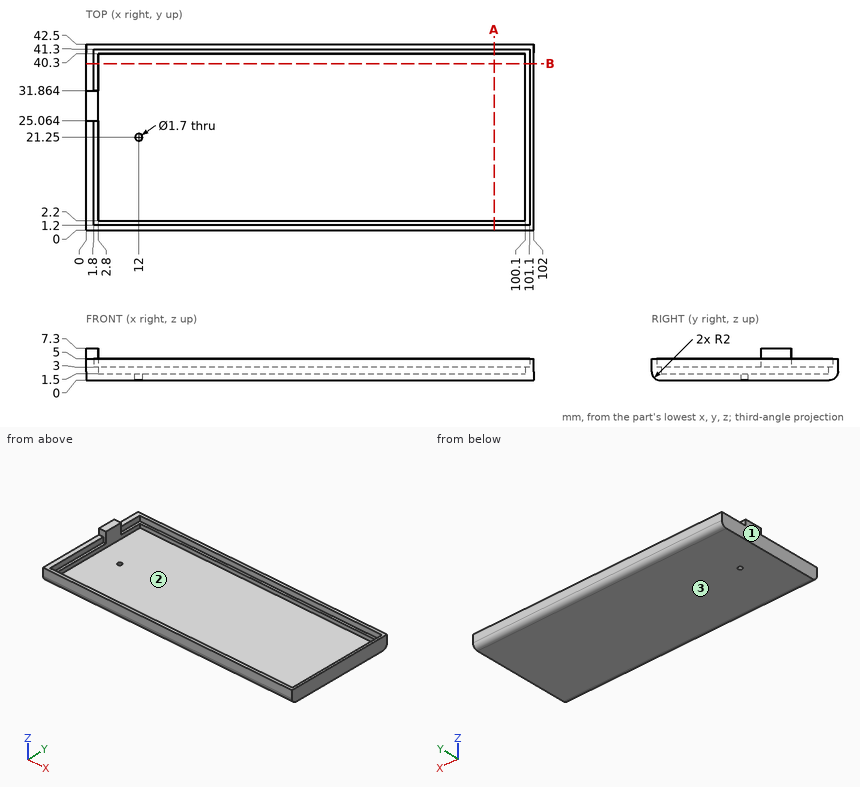
For this review, use the dimensioned drawing (mm, ordinates from the lowest corner) and the shaded views. Coordinates: 2 decimals unless noted, no trailing zeros. Write each loop counter-clockwise with the first axis right and the second up, starting at its lowest first coordinate (ties: lowest second). Pieces come first, ordered by that corner, then holes. Notation, with made-up numbers: (23.25, 81.25) - (71.25, 81.25) arc R23 ccw to (71.25, 92.25) - close; hole circle Ø3 at (-30.75, 9.5). An arc over 180 degrees is marked (long way). Answer in a Markdown table with one row per item. Add a question column.
Q1. Clearance check with a flat-ended pin moving along its axis: pin 1 (11.5 mm diameter, centred on x = 41, y = 16.5, fed in from +Z). State where the tip first meets the part, or that it passes through.
Q2. To check wall thickness, follow line 1 along Y through (x, z) = (24, 2.25); line 2 along Y through (x, z) = (29, 3.5); line 3 along X through (y, z) = (7.5, 3.5). State the ranges of each line that lie inside material, in increasing order. Write a range as from..to.
Q3. Draft analysis for pull direction X (two halves, no side actions). For the marked faces 1, 2 and 3, state which applies: +X half, -X half, draft (parallel to the pull), parting line (faces both ways), or undercut.
Q4. Consider section B-B on y = 38. Give the boundary of the cut face in (x, z).
Q5. Consider section A-A on x = 93. Give the boundary of the cut face in (y, z).
Answers below:
| question | item | result |
|---|---|---|
| 1 | pin 1 | z = 1.5 |
| 2 | line 1 | 0..2.2, 40.3..42.5 |
| 2 | line 2 | 0..1.2, 41.3..42.5 |
| 2 | line 3 | 0..1.8, 101.1..102 |
| 3 | face 1 | -X half |
| 3 | face 2 | undercut |
| 3 | face 3 | draft |
| 4 | outline | (0, 0) - (102, 0) - (102, 5) - (101.1, 5) - (101.1, 3) - (100.1, 3) - (100.1, 1.5) - (2.8, 1.5) - (2.8, 3) - (1.8, 3) - (1.8, 5) - (0, 5) - close |
| 5 | outline | (0, 2) arc R2 ccw to (2, 0) - (40.5, 0) arc R2 ccw to (42.5, 2) - (42.5, 5) - (41.3, 5) - (41.3, 3) - (40.3, 3) - (40.3, 1.5) - (2.2, 1.5) - (2.2, 3) - (1.2, 3) - (1.2, 5) - (0, 5) - close |
